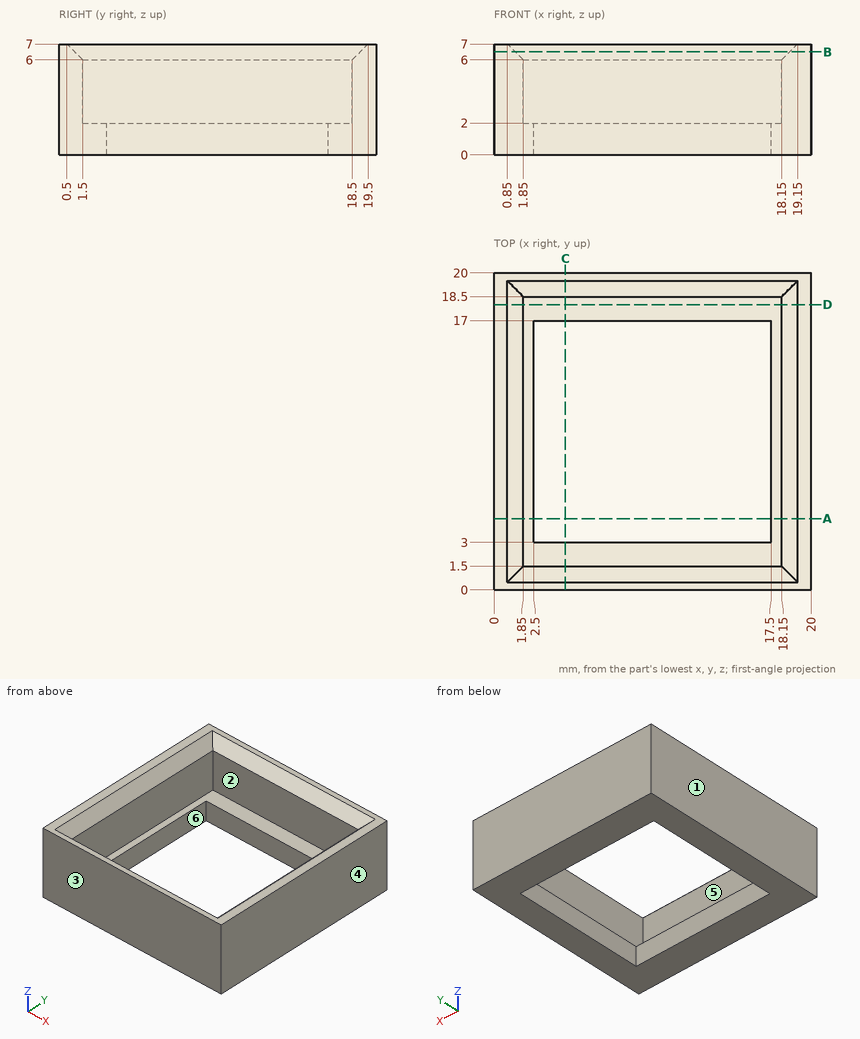
Could you check a few things on this drawing? It's one solid part, dimensions in mm from its lowest x, y, z. A direction names the side the tool comes from. Round coordinates to 2 decimals unless told otherwise and drop trailing zeros. Order: outer loops, then holes, each group sorted by start corner. A loop starts at its lowest first (then second) coordinate and runs counter-clockwise, first axis right, second up. Notation, with made-up numbers: M 80,60 L 111,60 A29 cw 111,84 Z; hole C 15,-10 d3. An arc over 180 degrees is marked long. One line per item, written item: value.
(1) I'm going to push flat-ended pins straight in: P1, Ø1, axis at y = 8.5, z = 3.5, coming from the -X side; P2, Ø3, axis at x = 5, y = 4, coming from the +Z side. Where does each tip first touch, or does it pass through?
Ans:
P1: stops at x = 0
P2: stops at z = 2
(2) I need wall thicknesses on line 1 along X through (y, z) = (15.75, 4.75); line 2 along Y through (x, z) = (12, 5); line 3 along X through (y, z) = (4.25, 0.5). Which ranges of each line are inside material? Lowest first, please. Write a range as from..to.
Ans:
line 1: x = 0..1.85, 18.15..20
line 2: y = 0..1.5, 18.5..20
line 3: x = 0..2.5, 17.5..20
(3) Imagine slicing it at B-B (z = 6.5). Write out the boundary of the cut face in (x, y).
Ans:
outline: M 0,0 L 20,0 L 20,20 L 0,20 Z; hole M 1.35,1 L 18.65,1 L 18.65,19 L 1.35,19 Z
(4) If we mould it in two halves opening along Y, with no side actions, what happens to the marked faces 1, 2 and 3? For each: released by +Y, released by -Y, zero draft, split by the parting line, or undercut.
Ans:
face 1: zero draft
face 2: undercut
face 3: released by -Y
(5) Imagine slicing it at D-D (y = 18). Write out the boundary of the cut face in (x, z).
Ans:
outline: M 0,0 L 20,0 L 20,7 L 19.15,7 L 18.15,6 L 18.15,2 L 1.85,2 L 1.85,6 L 0.85,7 L 0,7 Z
(6) Imagine slicing it at A-A (y = 4.5). Write out the boundary of the cut face in (x, z), and give its area (3 significant figures).
Ans:
outline: M 0,0 L 2.5,0 L 2.5,2 L 1.85,2 L 1.85,6 L 0.85,7 L 0,7 Z; M 17.5,0 L 20,0 L 20,7 L 19.15,7 L 18.15,6 L 18.15,2 L 17.5,2 Z
area: 27.5 mm^2
(7) Which directions (+Z, -Z, +X, -X, +Y, -Y) give clear straight access to the entire face, cutting with the end or side of a thin tool? Please do the marked faces 4, 5 and 6.
Ans:
face 4: +Z, -Z, +X, +Y, -Y
face 5: +Z
face 6: +Z, -Z
(8) Imagine slicing it at C-C (x = 4.5). Write out the boundary of the cut face in (y, z).
Ans:
outline: M 0,0 L 3,0 L 3,2 L 1.5,2 L 1.5,6 L 0.5,7 L 0,7 Z; M 17,0 L 20,0 L 20,7 L 19.5,7 L 18.5,6 L 18.5,2 L 17,2 Z
